Source: CAD feature listing. Evaluate the final solid. Frame: model axes, mm. A direction names the side the tool comes from. Round coordinates to 2 decimals unless told otherwise and drop trailing zeros. Loops run counter-clockwise (first coordinate to the right, second up) from the corner with the lowest first, then second, coordinate; pieces in that order, holes last. Notation, with made-up numbers: M -26,42.25 L -18,42.25 A15 cw -18,51.25 Z; hole C 58.5,13 d6. An arc over 180 degrees is marked long. Answer as a JSON object with one key per item and string values.
from build123d import *

# Parameters (mm, degrees)
SKETCH_1_R               = 7
EXTRUDE_1_DEPTH          = 5.1
SKETCH_4_R               = 0.95
CUT_EXTRUDE_2_DEPTH      = 8
SKETCH_5_R               = 5.6
SKETCH_5_R_2             = 2.15
CUT_EXTRUDE_3_DEPTH      = 4
SKETCH_6_W               = 3.7
SKETCH_6_H               = 0.8
CUT_EXTRUDE_4_DEPTH      = 4
CHAMFER_1_SIZE           = 0.8
CHAMFER_2_SIZE           = 0.8
SKETCH_7_R               = 1.5
CUT_EXTRUDE_5_DEPTH      = 0.4
SKETCH_8_R               = 0.9
CUT_EXTRUDE_6_DEPTH      = 5
CUT_EXTRUDE_6_DEPTH_BACK = 2.1


with BuildPart() as part:
    # Эскиз1 → Бобышка-Вытянуть1 (new body)
    with BuildSketch(Plane(origin=(0, 0, 0), x_dir=(1, 0, 0), z_dir=(0, 1, 0))):
        Circle(SKETCH_1_R)
    extrude(amount=EXTRUDE_1_DEPTH)

    # Эскиз4 → Вырез-Вытянуть2 (cut)
    with BuildSketch(Plane.XZ):
        Circle(SKETCH_4_R)
    extrude(amount=-CUT_EXTRUDE_2_DEPTH, mode=Mode.SUBTRACT)

    # Эскиз5 → Вырез-Вытянуть3 (cut)
    with BuildSketch(Plane(origin=(0, 0, 0), x_dir=(-1, 0, 0), z_dir=(0, -1, 0))):
        Circle(SKETCH_5_R)
        Circle(SKETCH_5_R_2, mode=Mode.SUBTRACT)
    extrude(amount=-CUT_EXTRUDE_3_DEPTH, mode=Mode.SUBTRACT)

    # Эскиз6 → Вырез-Вытянуть4 (cut)
    with BuildSketch(Plane.XZ):
        with Locations((0, 5.9)):
            Rectangle(SKETCH_6_W, SKETCH_6_H)
    extrude(amount=-CUT_EXTRUDE_4_DEPTH, mode=Mode.SUBTRACT)

    # Фаска1
    chamfer_1_edges = [part.edges().sort_by_distance(p)[0] for p in [
        (2.15, 0, 0),
    ]]
    chamfer(chamfer_1_edges, length=CHAMFER_1_SIZE)

    # Фаска2
    chamfer_2_edges = [part.edges().sort_by_distance(p)[0] for p in [
        (0, 0, -5.6),
    ]]
    chamfer(chamfer_2_edges, length=CHAMFER_2_SIZE)

    # Эскиз7 → Вырез-Вытянуть5 (cut)
    with BuildSketch(Plane.XZ.offset(-4)):
        with Locations((0, 4)):
            Circle(SKETCH_7_R)
        with Locations((3.464101615, -2)):
            Circle(SKETCH_7_R)
        with Locations((-3.464101615, -2)):
            Circle(SKETCH_7_R)
    extrude(amount=-CUT_EXTRUDE_5_DEPTH, mode=Mode.SUBTRACT)

    # Эскиз8 → Вырез-Вытянуть6 (cut, two sides)
    with BuildSketch(Plane.XZ.offset(-4)) as cut_extrude_6_sk:
        with Locations((0, 4)):
            Circle(SKETCH_8_R)
        with Locations((3.464101615, -2)):
            Circle(SKETCH_8_R)
        with Locations((-3.464101615, -2)):
            Circle(SKETCH_8_R)
    extrude(amount=CUT_EXTRUDE_6_DEPTH, mode=Mode.SUBTRACT)
    extrude(cut_extrude_6_sk.sketch, amount=-CUT_EXTRUDE_6_DEPTH_BACK, mode=Mode.SUBTRACT)


solid = part.part
Item 1: Section B-B on y = 1.7. Return the cut outline in (x, z), then the cut area to 3 significant figures.
Answer sheet:
{"outline": "C 0,0 d14; C 0,0 d4.3; hole M -1.85,5.5 L -1.05,5.5 A5.6 ccw long 1.05,5.5 L 1.85,5.5 L 1.85,6.3 L -1.85,6.3 Z; hole C 0,0 d1.9", "area": "64.3 mm²"}
Item 2: Section C-C on x = 0. Return the cut outline in (y, z).
Answer sheet:
{"outline": "M 0,-7 L 5.1,-7 L 5.1,-0.95 L 0,-0.95 L 0,-1.35 L 0.8,-2.15 L 4,-2.15 L 4,-5.6 L 0.8,-5.6 L 0,-6.4 Z; M 0,0.95 L 5.1,0.95 L 5.1,3.1 L 4.4,3.1 L 4.4,2.5 L 4,2.5 L 4,2.15 L 0.8,2.15 L 0,1.35 Z; M 0,6.3 L 4,6.3 L 4,5.5 L 4.4,5.5 L 4.4,4.9 L 5.1,4.9 L 5.1,7 L 0,7 Z"}
Item 3: Line query: probe 1 along Z at (x, y) = (0, 3.85); probe 2 along Y at (x, z) = (-2.5, 1.25); probe 3 along Z at (x, y) = (-0.75, 0.4). Output: solid intervals per line, ascending. Write a range as from..to.
Answer sheet:
{"probe 1": "z = -7..-5.6, -2.15..-0.95, 0.95..2.15, 6.3..7", "probe 2": "y = 4..5.1", "probe 3": "z = -6.96..-5.95, -1.58..-0.58, 0.58..1.58, 6.3..6.96"}
Item 4: Contact query for flat-ended pins moving along their axis: pin 1 Ø1.5 at (y, z) = (3, 4) entering from -X; pin 2 Ø1.5 at (x, z) = (3, -2) entering from -Y; pin 3 Ø1.5 at (x, z) = (0.5, -3.5) entering from -Y; pin 4 Ø1.4 at (x, z) = (0, 4) entering from -Y. Output: stop coordinate, or through.
Answer sheet:
{"pin 1": "stops at x = -6.2", "pin 2": "stops at y = 4.4", "pin 3": "stops at y = 4", "pin 4": "passes through"}
Item 5: Access query for faces 1 (the cylindrical face through (-0.195, 4.745, 3.121)), 2 (the cylindrical face through (-2.033, 4.197, -1.549)). Directions: +Z, -Z, +X, -X, +Y, -Y. A direction counts if a zero-diameter tool reaches every point of the face in a straight line with its end or side. Return the directions, or none.
Answer sheet:
{"face 1": "+Y, -Y", "face 2": "-Y"}
Item 6: Pull-direction query (X, two-part tool) for faces 3 (the cylindrical face through (2.8, 4.75, -1.39)), 4 (the cylindrical face through (6.466, 2.514, 2.681)), 5 (the flat face through (3, 0, 6)); classes: pulls with the +X half, pulls with the -X half, needs draft (parallel to the pull), parting line crosses it, or undercut.
Answer sheet:
{"face 3": "undercut", "face 4": "parting line crosses it", "face 5": "needs draft"}
Item 7: Section A-A on z = 0. Return the cut outline in (x, y), then the cut area to 3 significant figures.
Answer sheet:
{"outline": "M -7,0 L -6.4,0 L -5.6,0.8 L -5.6,4 L -2.15,4 L -2.15,0.8 L -1.35,0 L -0.95,0 L -0.95,5.1 L -7,5.1 Z; M 0.95,0 L 1.35,0 L 2.15,0.8 L 2.15,4 L 5.6,4 L 5.6,0.8 L 6.4,0 L 7,0 L 7,5.1 L 0.95,5.1 Z", "area": "32.8 mm²"}
